from build123d import *

# Parameters (mm, degrees)
F0_W     = 44.45
F0_H     = 25.4
F1_DEPTH = 25.4
F2_W     = 12.7
F2_H     = 12.7
F3_DEPTH = 6.35
F4_W     = 31.7093898326
F4_H     = 25.4
F5_DEPTH = 12.7
F7_DEPTH = 25.4
F8_R     = 6.2195299404
F9_DEPTH = 25.4


with BuildPart() as f1:
    # F0 (on Front) → F1 (new body)
    with BuildSketch(Plane.XZ):
        with Locations((22.225, 12.7)):
            Rectangle(F0_W, F0_H)
    extrude(amount=F1_DEPTH)

    # F2 (on face) → F3 (cut)
    with BuildSketch(Plane.XZ.offset(25.4)):
        with Locations((6.35, 12.7)):
            Rectangle(F2_W, F2_H)
    extrude(amount=-F3_DEPTH, mode=Mode.SUBTRACT)

    # F4 (on face) → F5 (cut)
    with BuildSketch(Plane.XZ.offset(25.4)):
        with Locations((28.5953050837, 12.7)):
            Rectangle(F4_W, F4_H)
    extrude(amount=-F5_DEPTH, mode=Mode.SUBTRACT)

    # F6 (on face) → F7 (cut)
    with BuildSketch(Plane.XZ.offset(12.7)):
        with BuildLine():
            Line((44.45, 25.4), (19.0906101674, 25.4))
            ThreePointArc((19.0906101674, 25.4), (31.7906101674, 12.7), (19.0906101674, 0))
            Line((19.0906101674, 0), (44.45, 0))
            Line((44.45, 0), (44.45, 25.4))
        make_face()
    extrude(amount=-F7_DEPTH, mode=Mode.SUBTRACT)

    # F8 (on face) → F9 (cut)
    with BuildSketch(Plane.XZ.offset(12.7)):
        with Locations((20.9586918354, 13.1910173222)):
            Circle(F8_R)
    extrude(amount=-F9_DEPTH, mode=Mode.SUBTRACT)


solid = f1.part
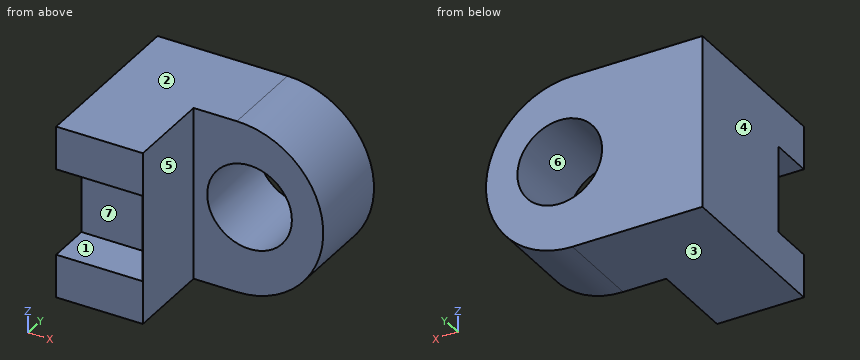
Here's how the part is built. I have some questions about the finished solid (model axes, mm). Face numbers are marked on the shaded views. A direction names the side the tool comes from. Round coordinates to 2 decimals unless told otherwise and drop trailing zeros. Order: outer loops, then holes, each group sorted by start corner. A loop starts at its lowest first (then second) coordinate and runs counter-clockwise, first axis right, second up. Notation, with made-up numbers: M -16,-18.75 L 20,-18.75 A15 ccw 20,2.25 Z; hole C 67.25,-36.5 d8. An arc over 180 degrees is marked long. Return JSON: item names as keys, results as strings. Group by question number.
1. Please list where these lines run through material, in increasing order: probe 1 along Z at (x, y) = (2, -20.25); probe 2 along X at (y, z) = (-13, 9.75); probe 3 along X at (y, z) = (-0.75, 10.5).
2. On a 3-axis mill with a long thin cutter (end or side, diameter ignored), from which of +Z, -Z, +X, -X, +Y, -Y can I reach the whole of each face in a straight line? I mean the marked faces 5, 6 and 7. Say none if no direction works.
3. If we section it at B-B on x = 17: List the corners of the cut face in (y, z) for me.
4. If we section it at D-D on y = -17: List the corners of the cut face in (x, z) for me, then the cut area to 3 significant figures.
5. If we section it at A-A on z = 17: List the corners of the cut face in (x, y) for me, then the cut area to 3 significant figures.
6. I'm going to push flat-ended pins straight in: pin 1 Ø6.5 at (x, z) = (6.5, 12) entering from -Y; pin 2 Ø3 at (y, z) = (-12, 20.5) entering from +X; pin 3 Ø5 at (y, z) = (-23.5, 13.5) entering from -X. Where does each tip first touch, or does it pass through?
7. If we mould it in two halves opening along Z, with no side actions, what happens to the marked faces 1, 2, 3 and 4? For each: pulls with the +Z half, pulls with the -Z half, needs draft (parallel to the pull), parting line crosses it, or undercut.
8. If we section it at C-C on x = 5: List the corners of the cut face in (y, z) for me.
Reply:
{
 "1": {"probe 1": "0 to 6.35, 19.05 to 25.4", "probe 2": "0 to 12.74", "probe 3": "0 to 15.35, 26.57 to 31.6"},
 "2": {"face 5": "+Z, -Z, +X, -Y", "face 6": "+Y, -Y", "face 7": "-X, -Y"},
 "3": {"outline": "M -12.7,0 L 0,0 L 0,8.39 L -12.7,8.39 Z; M -12.7,17.99 L 0,17.99 L 0,25.4 L -12.7,25.4 Z"},
 "4": {"outline": "M 0,0 L 12.74,0 L 12.74,25.4 L 0,25.4 Z", "area": "324 mm^2"},
 "5": {"outline": "M 0,-19.05 L 12.7,-19.05 L 12.7,-25.4 L 12.74,-25.4 L 12.74,-12.7 L 16.04,-12.7 L 16.04,0 L 0,0 Z; M 25.88,-12.7 L 31.04,-12.7 L 31.04,0 L 25.88,0 Z", "area": "350 mm^2"},
 "6": {"pin 1": "y = -19.05", "pin 2": "x = 30.12", "pin 3": "x = 12.7"},
 "7": {"face 1": "undercut", "face 2": "pulls with the +Z half", "face 3": "pulls with the -Z half", "face 4": "needs draft"},
 "8": {"outline": "M -25.4,0 L 0,0 L 0,25.4 L -25.4,25.4 L -25.4,19.05 L -19.05,19.05 L -19.05,6.35 L -25.4,6.35 Z"}
}
